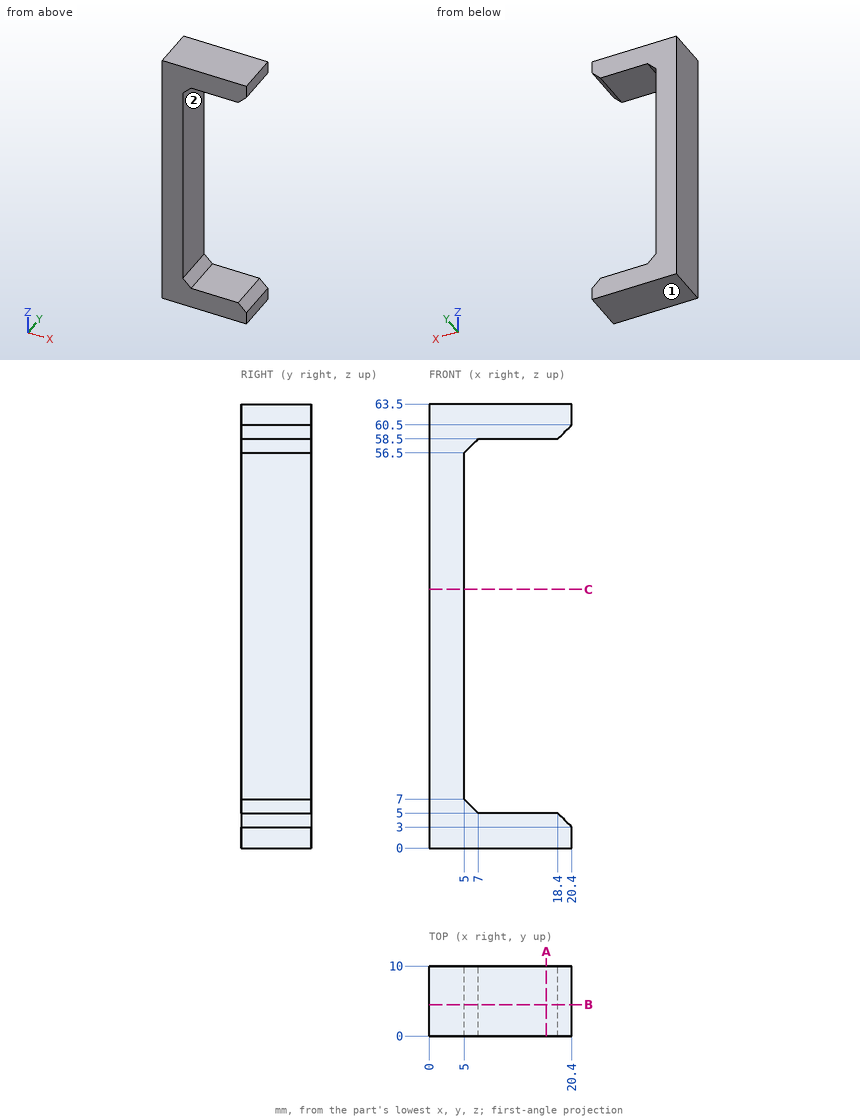
Could you check a few things on this drawing? It's one solid part, dimensions in mm from its lowest x, y, z. A direction names the side the tool comes from. Round coordinates to 2 decimals unless told otherwise and drop trailing zeros. Order: outer loops, then holes, each group sorted by start corner. A loop starts at its lowest first (then second) coordinate and runs counter-clockwise, first axis right, second up. Notation, with made-up numbers: (-3.5, 19.25) -> (35.5, 19.25) arc R21 cw to (35.5, 24.25) -> close; hole circle Ø9 at (58, -5). An arc over 180 degrees is marked (long way). One line per question, with ' | ' between items.
Q1. If I drill on line 1 (Z direction, x = 16.75, y = 6); line 2 (X direction, y = 7.5, z = 24.5); line 3 (Z direction, x = 19.75, y = 7.75), over which ranges is the centre line in solid material (lowest first)? Write a range as from..to.
Computed values:
line 1: 0..5, 58.5..63.5 | line 2: 0..5 | line 3: 0..3.65, 59.85..63.5
Q2. If we section it at B-B on y = 4.5: Write out the boundary of the cut face in (x, z), plus the area to 4 significant figures.
Computed values:
outline: (0, 0) -> (20.4, 0) -> (20.4, 3) -> (18.4, 5) -> (7, 5) -> (5, 7) -> (5, 56.5) -> (7, 58.5) -> (18.4, 58.5) -> (20.4, 60.5) -> (20.4, 63.5) -> (0, 63.5) -> close | area: 471.5 mm²
Q3. If we section it at A-A on x = 16.75: Write out the boundary of the cut face in (y, z), plus the area to 3 significant figures.
Computed values:
outline: (0, 0) -> (10, 0) -> (10, 5) -> (0, 5) -> close; (0, 58.5) -> (10, 58.5) -> (10, 63.5) -> (0, 63.5) -> close | area: 100 mm²
Q4. If we section it at C-C on z = 37: Write out the boundary of the cut face in (x, y).
Computed values:
outline: (0, 0) -> (5, 0) -> (5, 10) -> (0, 10) -> close
Q5. Which directions (+Z, -Z, +X, -X, +Y, -Y) give clear straight access to the entire face, cutting with the end or side of a thin tool? Please do the marked faces 1 and 2.
Computed values:
face 1: -Z, +X, -X, +Y, -Y | face 2: +X, +Y, -Y
Q6. I'm going to push flat-ended pins straight in: pin 1 (1 mm diameter, centred on y = 3.5, z = 43.5, fed in from -X); pin 2 (6 mm diameter, centred on y = 7, z = 50, fed in from +X). Where does each tip first touch, or does it pass through?
Computed values:
pin 1: x = 0 | pin 2: x = 5
